Autodesk Inventor part; units mm, degrees
ref_plane "YZ Plane" through (0, 0, 0) normal (1, 0, 0) x (0, 1, 0)
ref_plane "XZ Plane" through (0, 0, 0) normal (0, 1, 0) x (-1, 0, 0)
ref_plane "XY Plane" through (0, 0, 0) normal (0, 0, 1) x (1, 0, 0)
sketch "LEDT175, LED_28" plane through (0, 0, 0) normal (0, 0, 1) x (1, 0, 0)
  arc A0 (-2.794, -1.27) -> (0, -4.064) centre (0, -1.27) ccw
  arc A1 (0, -4.064) -> (2.794, -1.27) centre (0, -1.27) ccw
  arc A2 (2.794, -1.27) -> (1.7018, 1.3462) centre (-0.9101, -1.2803) ccw
  line L0 (1.7018, 1.3462) -> (-1.7018, 1.3462)
  arc A3 (-1.7018, 1.3462) -> (-2.794, -1.27) centre (0.9101, -1.2803) ccw
extrude "Extrusion1" add sketch "LEDT175, LED_28" along normal blind 3
properties part number "LED"
Design review of the part built by this model. Coordinates are the model's own, in mm. Give positions to 0.01 mm unless a question says otherwise; leave off trailing zeros. Order: outer loops, then holes, each group sorted by start corner. A loop starts at its lowest first (then second) coordinate and runs counter-clockwise, first axis right, second up. Notation, with made-up numbers: (75, -22.75) - (130, -22.75) arc R9 cw to (130, -10.75) - close; hole circle Ø11 at (-3.5, 55.5). An arc over 180 degrees is marked (long way). Use CSV: the item, a comma, the result in double quotes. Start each with the question number.
Q1. Take a section at B-B (x = -0.85). State the section outline as (y, z) points.
Q2. Take a section at A-A (z = 1.1). State the section outline as (x, y) points.
Q3. For line 1 (X direction, y = 0.35, z = 2.2); line 2 (X direction, y = -3, z = 0.2); line 3 (Y direction, x = 2.45, z = 2.5), list the stretches that pass through material, from the lowest coordinate up.
Q4. For P1, Ø1.5, axis at y = 0, z = 2.5, coming from the +X side, flat-tipped, find the tip position at first contact; note if it passes through.
Calculated:
1,outline,"(-3.93, 0) - (1.35, 0) - (1.35, 3) - (-3.93, 3) - close"
2,outline,"(-2.79, -1.27) arc R2.79 ccw to (2.79, -1.27) arc R3.7 ccw to (1.7, 1.35) - (-1.7, 1.35) arc R3.7 ccw to start"
3,line 1,"x = -2.42 to 2.42"
3,line 2,"x = -2.19 to 2.19"
3,line 3,"y = -2.61 to 0.28"
4,P1,"stops at x = 2.76"
